Geometry: see drawing. Coordinates: mm, zero at the bounding-box minimum. A direction names the side the tool comes from. Coordinates: 2 decimals unless noted, no trailing zeros. Loops run counter-clockwise (first coordinate to the right, second up) from the corner with the lowest first, then second, coordinate; pieces in that order, holes last. Notation, with made-up numbers: (-28, 71.25) - (24, 71.25) arc R25 cw to (24, 93.25) - close; hole circle Ø10 at (45, -37.75). An arc over 180 degrees is marked (long way). Use a Markdown table: item, result. Add a question column.
1. Ray query, L1, parallel to X at y = 16.5, z = 95.25 (3 decimals); L2, parallel to X at y = 23, z = 95; L3, parallel to Y at x = 92, z = 61.5. Return the intervals inside material, ascending. Write a range as [from, to].
2. Section query C-C on z = 95.25. Return the cut outline in (x, y) (3 decimals), then the cut area to 3 significant figures.
3. Section query B-B on y = 3. Return the cut outline in (x, z) (3 decimals), then the cut area to 3 significant figures.
4. Draft query along X for the marked faces 1, 2 and 3. Return one class per face: released by +X, released by -X, zero draft, split by the parting line, or undercut.
5. Contact query for flat-ended pins moving along their axis: P1, Ø1, axis at x = 55.5, z = 29.5, coming from the -Y side; P2, Ø4, axis at y = 37, z = 21.5, coming from the -X side; P3, Ø1.5, axis at y = 15, z = 68.5, coming from the +X side. Output: stop coordinate, or through.
6. Section query A-A on x = 95.25. Return the cut outline in (y, z) (3 decimals).
7. Section query D-D on y = 35.5. Return the cut outline in (x, z), then the cut area to 3 significant figures.
8. Access query for the marked faces 4 and 5. Directions: +Z, -Z, +X, -X, +Y, -Y. A direction counts if a zero-diameter tool reaches every point of the face in a straight line with its end or side. Return the directions, or none.
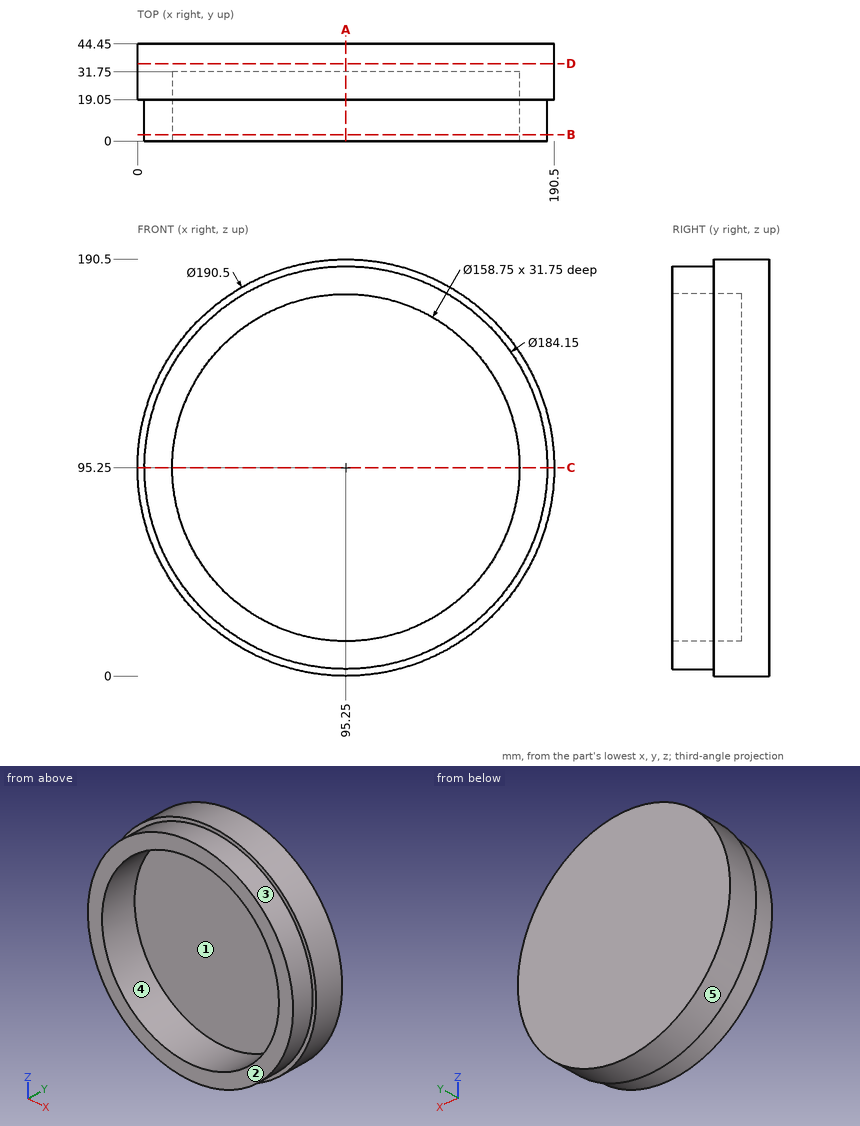
Resolved:
| question | item | result |
|---|---|---|
| 1 | L1 | [3.175, 15.875], [174.625, 187.325] |
| 1 | L2 | [0, 15.88], [174.62, 190.5] |
| 1 | L3 | [31.75, 44.45] |
| 2 | outline | (0, 19.05) - (3.175, 19.05) - (3.175, 0) - (15.875, 0) - (15.875, 31.75) - (174.625, 31.75) - (174.625, 0) - (187.325, 0) - (187.325, 19.05) - (190.5, 19.05) - (190.5, 44.45) - (0, 44.45) - close |
| 2 | area | 3,310 mm² |
| 3 | outline | circle Ø184.15 at (95.25, 95.25); hole circle Ø158.75 at (95.25, 95.25) |
| 3 | area | 6,840 mm² |
| 4 | face 1 | undercut |
| 4 | face 2 | zero draft |
| 4 | face 3 | split by the parting line |
| 5 | P1 | y = 31.75 |
| 5 | P2 | x = 32.6 |
| 5 | P3 | x = 183.58 |
| 6 | outline | (0, 3.175) - (19.05, 3.175) - (19.05, 0) - (44.45, 0) - (44.45, 190.5) - (19.05, 190.5) - (19.05, 187.325) - (0, 187.325) - (0, 174.625) - (31.75, 174.625) - (31.75, 15.875) - (0, 15.875) - close |
| 7 | outline | circle Ø190.5 at (95.25, 95.25) |
| 7 | area | 28,500 mm² |
| 8 | face 4 | -Y |
| 8 | face 5 | +Y, -Y |
